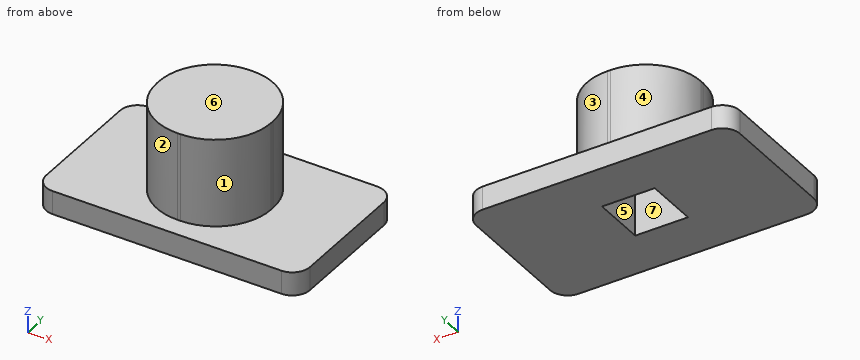
```python
from build123d import *

# Parameters (mm, degrees)
F0_W     = 9
F0_H     = 5.2
F1_DEPTH = 0.8
F2_W     = 3.9
F2_H     = 3.9
F3_DEPTH = 3
F4_R     = 1.9
F5_R     = 0.6
F6_W     = 1.8
F6_H     = 1.8
F7_DEPTH = 2.5


with BuildPart() as f1:
    # F0 (on Top) → F1 (new body)
    with BuildSketch(Plane.XY):
        Rectangle(F0_W, F0_H)
    extrude(amount=F1_DEPTH)

    # F2 (on face) → F3 (join)
    with BuildSketch(Plane.XY.offset(0.8)):
        Rectangle(F2_W, F2_H)
    extrude(amount=F3_DEPTH)

    # F4
    f4_edges = [f1.edges().sort_by_distance(p)[0] for p in [
        (-1.95, -1.95, 2.3),
        (-1.95, 1.95, 2.3),
        (1.95, -1.95, 2.3),
        (1.95, 1.95, 2.3),
    ]]
    fillet(f4_edges, radius=F4_R)

    # F5
    f5_edges = [f1.edges().sort_by_distance(p)[0] for p in [
        (-4.5, -2.6, 0.4),
        (-4.5, 2.6, 0.4),
        (4.5, -2.6, 0.4),
        (4.5, 2.6, 0.4),
    ]]
    fillet(f5_edges, radius=F5_R)

    # F6 (on face) → F7 (cut)
    with BuildSketch(Plane(origin=(0, 0, 0), x_dir=(1, 0, 0), z_dir=(0, 0, -1))):
        Rectangle(F6_W, F6_H)
    extrude(amount=-F7_DEPTH, mode=Mode.SUBTRACT)


solid = f1.part
```
Geometry check sheet. Reference: the model listing, model coordinates, mm. Face numbers are marked on the shaded views. A direction names the side the tool comes from. Round coordinates to 2 decimals unless told otherwise and drop trailing zeros. Order: outer loops, then holes, each group sorted by start corner. A loop starts at its lowest first (then second) coordinate and runs counter-clockwise, first axis right, second up. Notation, with made-up numbers: (37, 73.5) -> (46, 73.5) arc R24 cw to (46, 99.5) -> close; hole circle Ø3 at (62.25, 27.5). An arc over 180 degrees is marked (long way). Return JSON: item names as keys, results as strings. Group by question number.
Q1. Material ranges on probe 1 along Y at (x, z) = (0, 1.5); probe 2 along X at (y, z) = (-0.7, 0.25); probe 3 along Z at (x, y) = (-3.25, 0.05), recorded low to high. Write a range as from..to.
Q2. Gauge pin test, flat ends, axial feed: pin 1 (2 mm diameter, centred on x = 2, z = 2, fed in from +Y); pin 2 (1 mm diameter, centred on y = 1.5, z = 2.5, fed in from +X); pin 3 (1.5 mm diameter, centred on y = 1.5, z = 2, fed in from +X). Record the tip position at first contact, or that the pin passes through.
Q3. Release check for a two-part mould opening along X. For the marked faces 4, 5, 6 and 7 record: released by +X, released by -X, zero draft, split by the parting line, or undercut.
Q4. Section check A-A, the plane z = 0.45. Record the boundary of the cut face in (x, y), plus the area to 3 significant figures.
Q5. Section check D-D, the plane z = 3.2. Record the boundary of the cut face in (x, y).
Q6. Section check B-B, the plane z = 1.9. Record the boundary of the cut face in (x, y).
Q7. Tool access check on the marked faces 1, 2 and 3. Record the directions out of +Z, -Z, +X, -X, +Y, -Y that give a thin tool (end or side, any length) a straight path to the whole face; none if there is none.
Q8. Section check C-C, the plane x = -0.25. Record the boundary of the cut face in (y, z).
Numbers:
{
 "1": {"probe 1": "-1.95..-0.9, 0.9..1.95", "probe 2": "-4.5..-0.9, 0.9..4.5", "probe 3": "0..0.8"},
 "2": {"pin 1": "y = 1.7", "pin 2": "x = 1.7", "pin 3": "x = 1.82"},
 "3": {"face 4": "released by -X", "face 5": "undercut", "face 6": "zero draft", "face 7": "undercut"},
 "4": {"outline": "(-4.5, -2) arc R0.6 ccw to (-3.9, -2.6) -> (3.9, -2.6) arc R0.6 ccw to (4.5, -2) -> (4.5, 2) arc R0.6 ccw to (3.9, 2.6) -> (-3.9, 2.6) arc R0.6 ccw to (-4.5, 2) -> close; hole (-0.9, -0.9) -> (0.9, -0.9) -> (0.9, 0.9) -> (-0.9, 0.9) -> close", "area": "43.3 mm^2"},
 "5": {"outline": "(-1.95, -0.05) arc R1.9 ccw to (-0.05, -1.95) -> (0.05, -1.95) arc R1.9 ccw to (1.95, -0.05) -> (1.95, 0.05) arc R1.9 ccw to (0.05, 1.95) -> (-0.05, 1.95) arc R1.9 ccw to (-1.95, 0.05) -> close"},
 "6": {"outline": "(-1.95, -0.05) arc R1.9 ccw to (-0.05, -1.95) -> (0.05, -1.95) arc R1.9 ccw to (1.95, -0.05) -> (1.95, 0.05) arc R1.9 ccw to (0.05, 1.95) -> (-0.05, 1.95) arc R1.9 ccw to (-1.95, 0.05) -> close; hole (-0.9, -0.9) -> (0.9, -0.9) -> (0.9, 0.9) -> (-0.9, 0.9) -> close"},
 "7": {"face 1": "+Z, +X, -Y", "face 2": "+Z, -X, -Y", "face 3": "+Z, +X, +Y"},
 "8": {"outline": "(-2.6, 0) -> (-0.9, 0) -> (-0.9, 2.5) -> (0.9, 2.5) -> (0.9, 0) -> (2.6, 0) -> (2.6, 0.8) -> (1.94, 0.8) -> (1.94, 3.8) -> (-1.94, 3.8) -> (-1.94, 0.8) -> (-2.6, 0.8) -> close"}
}
